Autodesk Fusion 360 part; units mm, degrees
sketch "Sketch1" plane through (0, 0, 0) normal (0, 0, 1) x (1, 0, 0)
  line L0 (0, 0) -> (98, 0)
  line L1 (98, 0) -> (98, 98)
  line L2 (98, 98) -> (0, 98)
  line L3 (0, 98) -> (0, 0)
extrude "Extrude1" add sketch "Sketch1" along normal blind 5
sketch "Sketch2" plane through (0, 0, 0) normal (0, 0, 1) x (1, 0, 0)
  circle A0 centre (7.75, 7.75) radius 2.1
extrude "Extrude2" cut sketch "Sketch2" along normal blind 5
sketch "Sketch3" plane through (0, 0, 0) normal (0, 0, 1) x (1, 0, 0)
  circle A0 centre (7.75, 90.25) radius 2.1
extrude "Extrude3" cut sketch "Sketch3" along normal blind 5
sketch "Sketch4" plane through (0, 0, 0) normal (0, 0, 1) x (1, 0, 0)
  circle A0 centre (90.25, 7.75) radius 2.1
extrude "Extrude4" cut sketch "Sketch4" along normal blind 5
sketch "Sketch5" plane through (0, 0, 0) normal (0, 0, 1) x (1, 0, 0)
  circle A0 centre (90.25, 90.25) radius 2.1
extrude "Extrude5" cut sketch "Sketch5" along normal blind 5
sketch "Sketch6" plane through (0, 0, 0) normal (0, 0, 1) x (1, 0, 0)
  circle A0 centre (49, 49) radius 25
extrude "Extrude6" cut sketch "Sketch6" along normal blind 5
sketch "Sketch7" plane through (0, 0, 0) normal (0, 0, 1) x (1, 0, 0)
  line L0 (13, 14) -> (19, 14)
  line L1 (19, 14) -> (19, 84)
  line L2 (19, 84) -> (13, 84)
  line L3 (13, 84) -> (13, 14)
extrude "Extrude7" cut sketch "Sketch7" along normal blind 5
sketch "Sketch8" plane through (0, 0, 0) normal (0, 0, 1) x (1, 0, 0)
  line L0 (23, 14) -> (29, 14)
  line L1 (29, 14) -> (29, 84)
  line L2 (29, 84) -> (23, 84)
  line L3 (23, 84) -> (23, 14)
extrude "Extrude8" cut sketch "Sketch8" along normal blind 5
sketch "Sketch9" plane through (0, 0, 0) normal (0, 0, 1) x (1, 0, 0)
  line L0 (33, 14) -> (39, 14)
  line L1 (39, 14) -> (39, 84)
  line L2 (39, 84) -> (33, 84)
  line L3 (33, 84) -> (33, 14)
extrude "Extrude9" cut sketch "Sketch9" along normal blind 5
sketch "Sketch10" plane through (0, 0, 0) normal (0, 0, 1) x (1, 0, 0)
  line L0 (59, 14) -> (65, 14)
  line L1 (65, 14) -> (65, 84)
  line L2 (65, 84) -> (59, 84)
  line L3 (59, 84) -> (59, 14)
extrude "Extrude10" cut sketch "Sketch10" along normal blind 5
sketch "Sketch11" plane through (0, 0, 0) normal (0, 0, 1) x (1, 0, 0)
  line L0 (69, 14) -> (75, 14)
  line L1 (75, 14) -> (75, 84)
  line L2 (75, 84) -> (69, 84)
  line L3 (69, 84) -> (69, 14)
extrude "Extrude11" cut sketch "Sketch11" along normal blind 5
sketch "Sketch12" plane through (0, 0, 0) normal (0, 0, 1) x (1, 0, 0)
  line L0 (79, 14) -> (85, 14)
  line L1 (85, 14) -> (85, 84)
  line L2 (85, 84) -> (79, 84)
  line L3 (79, 84) -> (79, 14)
extrude "Extrude12" cut sketch "Sketch12" along normal blind 5
Read the model definition and answer for the solid it produces. Units are mm, in the model's axes. A direction names the side the tool comes from. Coordinates: 2 decimals unless noted, no trailing zeros. Write each loop counter-clockwise with the first axis right and the second up, starting at its lowest first coordinate (ties: lowest second). Pieces come first, ordered by that corner, then holes. Notation, with made-up numbers: (55.5, 36) -> (94.5, 36) arc R29 ccw to (94.5, 58) -> close; hole circle Ø8 at (-39, 21). An arc over 180 degrees is marked (long way). Answer as a JSON object with one key per item and string values.
Q1. A tool of negligible diameter and unlimited length cuts with its end or side. For faces 5 (the flat face through (82, 14, 2)), 6 (the flat face through (98, 48, 2)), from which of +Z, -Z, +X, -X, +Y, -Y can it reach the whole face along a straight path? Write none if from no direction.
The answers:
{"face 5": "+Z, -Z", "face 6": "+Z, -Z, +X, +Y, -Y"}
Q2. Consider line 1 (Y direction, x = 7.75, z = 3.1); line 2 (X direction, y = 37, z = 2.5); line 3 (Y direction, x = 15.5, z = 1.35). Determine where each line is inside the solid, lowest interval first. Write a range as [from, to].
The answers:
{"line 1": "y = [0, 5.65], [9.85, 88.15], [92.35, 98]", "line 2": "x = [0, 13], [19, 23], [75, 79], [85, 98]", "line 3": "y = [0, 14], [84, 98]"}
Q3. The part is cut by section A-A on y = 90.25. Give the vertices of the cut face in (x, z), then the cut area to 3 significant figures.
The answers:
{"outline": "(0, 0) -> (5.65, 0) -> (5.65, 5) -> (0, 5) -> close; (9.85, 0) -> (88.15, 0) -> (88.15, 5) -> (9.85, 5) -> close; (92.35, 0) -> (98, 0) -> (98, 5) -> (92.35, 5) -> close", "area": "448 mm2"}
Q4. The part is cut by section B-B on x = 17. Give the vertices of the cut face in (y, z).
The answers:
{"outline": "(0, 0) -> (14, 0) -> (14, 5) -> (0, 5) -> close; (84, 0) -> (98, 0) -> (98, 5) -> (84, 5) -> close"}
Q5. Determine the mould class of faces 1 (the flat face through (48, 82, 0)), 2 (the flat face through (69, 74, 2)), 3 (the flat face through (48, 0, 2)), 4 (the flat face through (85, 49, 2)) for opening direction Y: pulls with the +Y half, pulls with the -Y half, needs draft (parallel to the pull), parting line crosses it, or undercut.
The answers:
{"face 1": "needs draft", "face 2": "undercut", "face 3": "pulls with the -Y half", "face 4": "undercut"}
Q6. The part is cut by section C-C on y = 49.5. Give the vertices of the cut face in (x, z).
The answers:
{"outline": "(0, 0) -> (13, 0) -> (13, 5) -> (0, 5) -> close; (19, 0) -> (23, 0) -> (23, 5) -> (19, 5) -> close; (75, 0) -> (79, 0) -> (79, 5) -> (75, 5) -> close; (85, 0) -> (98, 0) -> (98, 5) -> (85, 5) -> close"}
Q7. A flat-ended cylindrical pin translates along its axis: pin 1 Ø2.5 at (x, z) = (37, 2) entering from -Y. Find the tip coordinate at first contact, or state that the pin passes through.
The answers:
{"pin 1": "stops at y = 0"}
